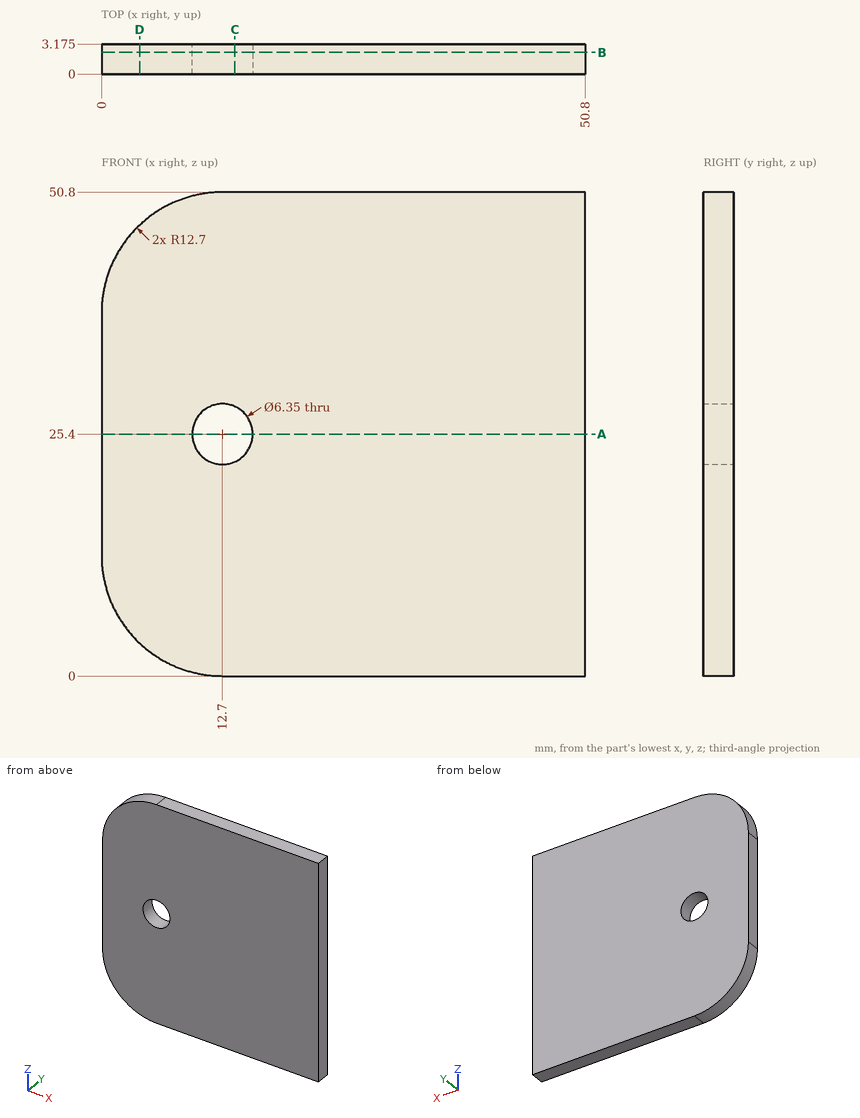
The figure shows three views and two pictorial views of one solid part (mm, origin at its lowest corner). Answer the questions. Give positions to 0.01 mm unless a question says otherwise; leave off trailing zeros. Order: outer loops, then holes, each group sorted by start corner. A loop starts at its lowest first (then second) coordinate and runs counter-clockwise, first axis right, second up. Notation, with made-up numbers: (32.5, 51.5) -> (70.5, 51.5) arc R13 cw to (70.5, 63.5) -> close; hole circle Ø8 at (75, -33). An arc over 180 degrees is marked (long way). Answer as a JSON object with one key per item and string values. Group by question number.
Item 1: The part is cut by section C-C on x = 14. Write down the section's boundary in (y, z) (3 decimals), and give its area (3 significant figures).
Item 2: The part is cut by section B-B on y = 2.3. Write down the section's boundary in (x, z) (3 decimals), and give its area (3 significant figures).
Item 3: The part is cut by section D-D on x = 4. Write down the section's boundary in (y, z) (3 decimals).
Item 4: Consider L1, parallel to Z at x = 12.7, y = 1.5 (3 decimals); L2, parallel to X at y = 1.45, z = 40; L3, parallel to X at y = 0.6, z = 9. Determine where each line is inside the solid, lowest interval first. Write a range as from..to.
Item 5: A flat-ended cylindrical pin translates along its axis: pin 1 (1 mm diameter, centred on x = 7.5, z = 31, fed in from -Y). Find the tip coordinate at first contact, or state that the pin passes through.
Item 6: The part is cut by section A-A on z = 25.4. Write down the section's boundary in (x, y) (3 decimals).
Result set:
{
 "1": {"outline": "(0, 0) -> (3.175, 0) -> (3.175, 22.503) -> (0, 22.503) -> close; (0, 28.297) -> (3.175, 28.297) -> (3.175, 50.8) -> (0, 50.8) -> close", "area": "143 mm²"},
 "2": {"outline": "(0, 12.7) arc R12.7 ccw to (12.7, 0) -> (50.8, 0) -> (50.8, 50.8) -> (12.7, 50.8) arc R12.7 ccw to (0, 38.1) -> close; hole circle Ø6.35 at (12.7, 25.4)", "area": "2,480 mm²"},
 "3": {"outline": "(0, 3.448) -> (3.175, 3.448) -> (3.175, 47.352) -> (0, 47.352) -> close"},
 "4": {"L1": "0..22.225, 28.575..50.8", "L2": "0.14..50.8", "L3": "0.55..50.8"},
 "5": {"pin 1": "y = 0"},
 "6": {"outline": "(0, 0) -> (9.525, 0) -> (9.525, 3.175) -> (0, 3.175) -> close; (15.875, 0) -> (50.8, 0) -> (50.8, 3.175) -> (15.875, 3.175) -> close"}
}
